Check sheet for the modelled part. Datum: model origin and axes. Units: mm. Face numbers are marked on the shaded views. Round coordinates to 2 decimals unless told otherwise and drop trailing zeros. Loops run counter-clockwise (first coordinate to the right, second up) from the corner with the lowest first, then second, coordinate; pieces in that order, holes last. Notation, with made-up numbers: (47, 51.25) - (105, 51.25) arc R24 cw to (105, 87.25) - close; hole circle Ø3 at (16.5, 57.5). An arc over 180 degrees is marked (long way). Return JSON: item names as keys, results as strings.
from build123d import *

# Parameters (mm, degrees)
F0_W     = 150
F0_H     = 20
F1_DEPTH = 4
F2_R     = 5
F3_DEPTH = 100
F4_R     = 5


with BuildPart() as f1:
    # F0 (on Front) → F1 (new body)
    with BuildSketch(Plane.XZ):
        with Locations((0.326128, -57.731088)):
            Rectangle(F0_W, F0_H)
    extrude(amount=F1_DEPTH)

    # F2 (on face) → F3 (join)
    with BuildSketch(Plane.XZ.offset(4)):
        with Locations((68.326128, -57.731088)):
            Circle(F2_R)
        with Locations((-67.673872, -57.731088)):
            Circle(F2_R)
    extrude(amount=F3_DEPTH)

    # F4
    f4_edges = [f1.edges().sort_by_distance(p)[0] for p in [
        (-74.673872, -2, -67.731088),
        (-74.673872, -2, -47.731088),
        (75.326128, -2, -67.731088),
        (75.326128, -2, -47.731088),
    ]]
    fillet(f4_edges, radius=F4_R)


solid = f1.part
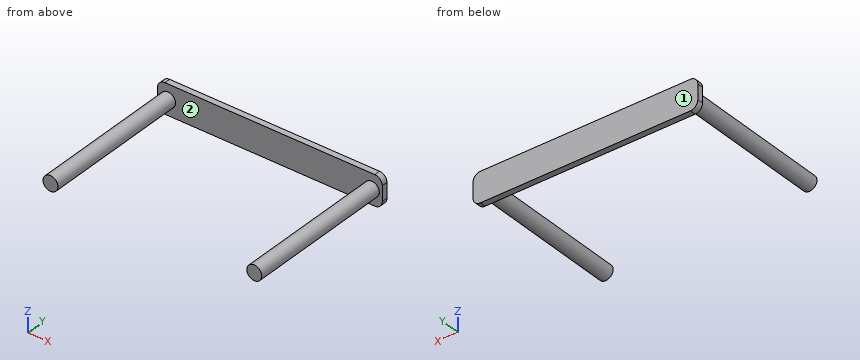
Q1. Scan lines: probe 1 along X at (y, z) = (-14, -57.75); probe 2 along Y at (x, z) = (-55, -64.75); probe 3 along X at (y, z) = (-86, -53.75). Record each from-to range of solid material in increasing order. Write a range as [from, to].
Answer key:
{"probe 1": "x = [-72.67, -62.67], [63.33, 73.33]", "probe 2": "y = [-4, 0]", "probe 3": "x = [-70.7, -64.65], [65.3, 71.35]"}
Q2. Sectioned sample at D-D (z = -49.5). Enter the section's corners in (x, y).
Answer key:
{"outline": "(-73.49, -4) - (74.14, -4) - (74.14, 0) - (-73.49, 0) - close"}
Q3. Sectioned sample at C-C (y = -23.5). Enter the section's corners in (x, z).
Answer key:
{"outline": "circle Ø10 at (-67.67, -57.73); circle Ø10 at (68.33, -57.73)"}
Q4. Sectioned sample at B-B (x = -32.5). Enter the section's corners in (y, z), plus the area to 3 significant figures.
Answer key:
{"outline": "(-4, -67.73) - (0, -67.73) - (0, -47.73) - (-4, -47.73) - close", "area": "80.0 mm²"}
Q5. Depth check by flat-ended pin: P1, Ø3, axis at x = 25.5, z = -57.5, coming from the -Y side; P2, Ø2, axis at y = -82.5, z = -53.5, coming from the -X side; P3, Ø8, axis at y = -72.5, z = -62, coming from the -X side. Enter the tip coordinate at first touch or a pass-through.
Answer key:
{"P1": "stops at y = -4", "P2": "stops at x = -71.49", "P3": "stops at x = -72.67"}
Q6. Sectioned sample at A-A (z = -59.5). Enter the section's corners in (x, y), plus the area to 3 significant figures.
Answer key:
{"outline": "(-74.67, -4) - (-72.35, -4) - (-72.35, -104) - (-63, -104) - (-63, -4) - (63.65, -4) - (63.65, -104) - (73, -104) - (73, -4) - (75.33, -4) - (75.33, 0) - (-74.67, 0) - close", "area": "2,470 mm²"}
Q7. Draft check along X on the marked faces 1 and 2. Enter one of: released by +X, released by -X, zero draft, split by the parting line, or undercut.
Answer key:
{"face 1": "zero draft", "face 2": "undercut"}
